Source: three-view drawing plus pictorial views. Frame: mm from the lowest corner of the part. Give positions to 0.01 mm unless a question says otherwise; leave off trailing zeros. Order: outer loops, then holes, each group sorted by start corner. A loop starts at its lowest first (then second) coordinate and runs counter-clockwise, first axis right, second up. Notation, with made-up numbers: (-36.5, 80) - (-16.5, 80) arc R36 ccw to (-16.5, 118) - close; hole circle Ø4 at (58.25, 3). An arc over 180 degrees is marked (long way). Answer in a Markdown table with one row per item. Add a question column.
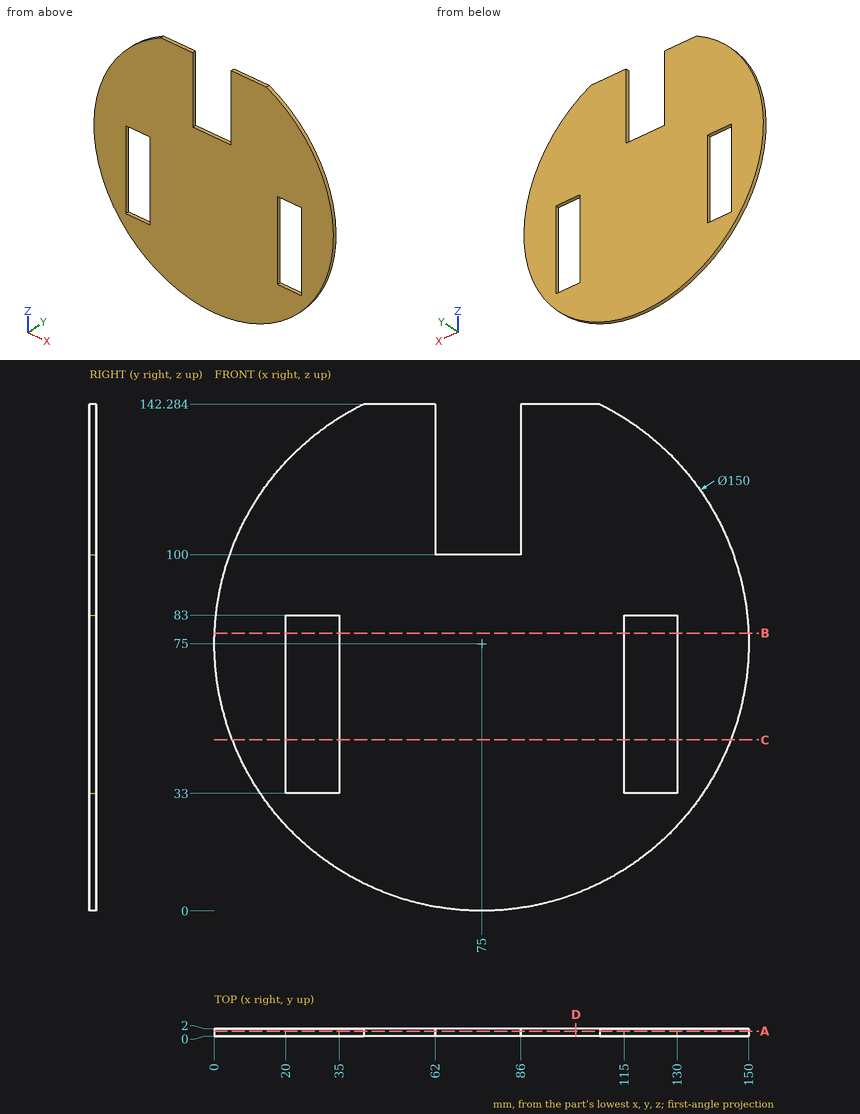
Q1. Section D-D, the plane x = 101.5. Return loops of the section in (y, z), then the cut area to 3 significant figures.
Q2. Contact query for flat-ended pins moving along their axis: P1, Ø1, axis at x = 123, y = 1, coming from the +Z side; P2, Ø0.6, axis at x = 27.5, y = 1, coming from the +Z side (1 decimal); P3, Ø1, axis at y = 1.5, z = 50, coming from the -X side (1 decimal). Output: stop coordinate, or through.
Q3. Line query: probe 1 along X at (y, z) = (1.4, 74.5); probe 2 along Z at (x, y) = (126, 0.5); probe 3 along X at (y, z) = (1.8, 70.5) (1 decimal). Output: solid intervals per line, ascending.
Q4. Section A-A, the plane y = 1.35. Return loops of the section in (x, z), then the cut area to 3 significant figures.
Q5. Section B-B, the plane z = 78. Return loops of the section in (x, y).
Q6. Section C-C, the plane z = 48. Return loops of the section in (x, y).
Computed:
| question | item | result |
|---|---|---|
| 1 | outline | (0, 4.84) - (2, 4.84) - (2, 142.28) - (0, 142.28) - close |
| 1 | area | 275 mm^2 |
| 2 | P1 | stops at z = 133.04 |
| 2 | P2 | stops at z = 133.3 |
| 2 | P3 | stops at x = 4.1 |
| 3 | probe 1 | x = 0 to 20, 35 to 115, 130 to 150 |
| 3 | probe 2 | z = 20.01 to 33, 83 to 129.99 |
| 3 | probe 3 | x = 0.1 to 20, 35 to 115, 130 to 149.9 |
| 4 | outline | (41.87, 142.28) arc R75 ccw (long way) to (108.13, 142.28) - (86, 142.28) - (86, 100) - (62, 100) - (62, 142.28) - close; hole (20, 33) - (35, 33) - (35, 83) - (20, 83) - close; hole (115, 33) - (130, 33) - (130, 83) - (115, 83) - close |
| 4 | area | 14,800 mm^2 |
| 5 | outline | (0.06, 0) - (20, 0) - (20, 2) - (0.06, 2) - close; (35, 0) - (115, 0) - (115, 2) - (35, 2) - close; (130, 0) - (149.94, 0) - (149.94, 2) - (130, 2) - close |
| 6 | outline | (5.03, 0) - (20, 0) - (20, 2) - (5.03, 2) - close; (35, 0) - (115, 0) - (115, 2) - (35, 2) - close; (130, 0) - (144.97, 0) - (144.97, 2) - (130, 2) - close |
